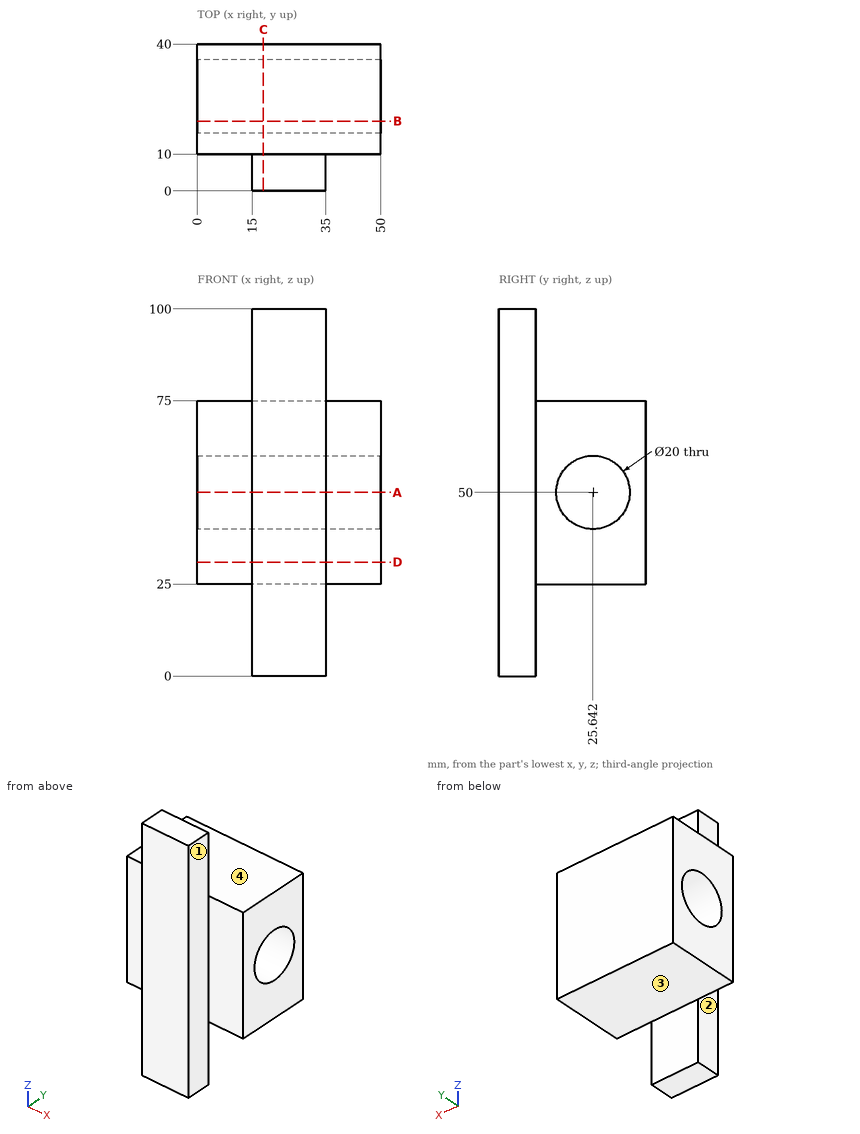
Input: dimensioned drawing with shaded views. Units: mm. Origin: part minimum x, y, z. A direction names the side the tool comes from. Round coordinates to 2 decimals unless told otherwise and drop trailing zeros. Loops run counter-clockwise (first coordinate to the right, second up) from the corner with the lowest first, then second, coordinate; pieces in that order, holes last. Notation, with made-up numbers: (24, -13.5) -> (69, -13.5) arc R24 ccw to (69, 25.5) -> close; hole circle Ø8 at (6.25, 22). An arc over 180 degrees is marked (long way). One line per item, written item: value.
(1) Section A-A (z = 50). Return the cut outline in (x, y), plus the area to 3 significant figures.
Geometry check:
outline: (0, 10) -> (15, 10) -> (15, 0) -> (35, 0) -> (35, 10) -> (50, 10) -> (50, 15.64) -> (0, 15.64) -> close; (0, 35.64) -> (50, 35.64) -> (50, 40) -> (0, 40) -> close
area: 700 mm2
(2) Pin query (flat end, axial travel): pin 1 (24 mm diameter, centred on x = 30, y = 29.5, fed in from +Z); pin 2 (10 mm diameter, centred on x = 23, z = 8.5, fed in from +Y); pin 3 (4 mm diameter, centred on x = 22, y = 12.5, fed in from -Z). Return the tip coordinate at first contact, or that it passes through.
Geometry check:
pin 1: z = 75
pin 2: y = 10
pin 3: z = 25
(3) Section C-C (x = 18). Return the cut outline in (y, z).
Geometry check:
outline: (0, 0) -> (10, 0) -> (10, 25) -> (40, 25) -> (40, 75) -> (10, 75) -> (10, 100) -> (0, 100) -> close; hole circle Ø20 at (25.64, 50)
(4) Section D-D (z = 31). Return the cut outline in (x, y).
Geometry check:
outline: (0, 10) -> (15, 10) -> (15, 0) -> (35, 0) -> (35, 10) -> (50, 10) -> (50, 40) -> (0, 40) -> close
(5) Material intervals for line 1 (Y direction, x = 23, z = 50); line 2 (Y direction, x = 14, z = 50); line 3 (Y direction, x = 40, z = 38.5), sorted ascending. Write a range as [from, to].
Geometry check:
line 1: [0, 15.64], [35.64, 40]
line 2: [10, 15.64], [35.64, 40]
line 3: [10, 40]
(6) Section B-B (y = 19). Return the cut outline in (x, z).
Geometry check:
outline: (0, 25) -> (50, 25) -> (50, 42.52) -> (0, 42.52) -> close; (0, 57.48) -> (50, 57.48) -> (50, 75) -> (0, 75) -> close
(7) Set-up query: the marked faces 1, 2, 3 and 4. Return all of +Z, -Z, +X, -X, +Y, -Y with unobstructed straight access to the full face (end or side cutting, diameter ignored); none if empty.
Geometry check:
face 1: +Z, -Z, +X, -Y
face 2: +Z, -Z, -X, -Y
face 3: -Z, +X, -X, +Y
face 4: +Z, +X, -X, +Y
